Autodesk Inventor part; units mm, degrees
ref_plane "YZ Plane" through (0, 0, 0) normal (1, 0, 0) x (0, 1, 0)
ref_plane "XZ Plane" through (0, 0, 0) normal (0, 1, 0) x (-1, 0, 0)
ref_plane "XY Plane" through (0, 0, 0) normal (0, 0, 1) x (1, 0, 0)
sketch "Эскиз1" plane through (0, 0, 0) normal (1, 0, 0) x (0, 1, 0)
  circle A0 centre (0, 0) radius 4
  circle A1 centre (0, 0) radius 5
  line L0 (0, 5) -> (-2, 5)
  line L1 (-2, 5) -> (-2, 10)
  line L2 (-2, 10) -> (0, 10)
  line L3 (0, 10) -> (0, 5)
  line L4 (0, -5) -> (-2, -5)
  line L5 (-2, -5) -> (-2, -10)
  line L6 (-2, -10) -> (0, -10)
  line L7 (0, -10) -> (0, -5)
  line L8 (-2, 5) -> (-2, -5)
  line L9 (0, 5) -> (-2, 4.5826)
  line L10 (-2, -4.5826) -> (0, -5)
  line L11 (-2, 2) -> (-1, 3.873)
  line L12 (-2, -2) -> (-1, -3.873)
  line L13 (-1, -3.873) -> (-2, -3.873)
  line L14 (-1, 3.873) -> (-2, 3.873)
  dimension "d0" = 8
  dimension "d1" = 10
  dimension "d2" = 3
  dimension "d3" = 3
extrude "Выдавливание1" add sketch "Эскиз1" along normal blind 8 contours A0 L14 L8 L9 A1 L10 L13 | L11 L8 A0 | A0 L8 L14 | L13 L8 A0 | A0 L8 L12 | L8 L0 A1 | A1 L9 | L10 A1 | A1 L4 L8 | L0 L1 L2 L3 | L7 L6 L5 L4
fillet "Сопряжение2" radius 1.25 2 edges at (4, 0, 10) (4, 0, -10)
fillet "Сопряжение3" radius 1.5 2 edges at (4, -1, -3.873) (4, -1, 3.873)
sketch "Эскиз5" plane through (8, 0, 0) normal (1, 0, 0) x (0, 0, -1)
  circle A0 centre (0, 0) radius 5
  circle A1 centre (0, 0) radius 6
  line L0 (-5, 0) -> (-8.75, 0)
  line L1 (-6, 0) -> (-5, 0)
  arc A2 (5, 0) -> (-5, 0) centre (0, 0) ccw
  line L2 (-5, 0) -> (5, 0)
  line L3 (8.75, 0) -> (5, 0)
  line L4 (6, 0) -> (5, 0)
  dimension "d28" = 12
extrude "Выдавливание5" add sketch "Эскиз5" against normal blind 8 contours A0 L0 A1 L3 picked at (-5.5601, 0.8775)
fillet "Сопряжение4" radius 2.5 2 edges at (4, 0, 6) (4, 0, -6)
properties part number "binding links"
Verification items for the finished model (mm, model axes). A direction names the side the tool comes from. Round coordinates to 2 decimals unless told otherwise and drop trailing zeros. Order: outer loops, then holes, each group sorted by start corner. A loop starts at its lowest first (then second) coordinate and runs counter-clockwise, first axis right, second up. Notation, with made-up numbers: (49.5, 22.5) -> (65.5, 22.5) arc R26 ccw to (65.5, 46.5) -> close; hole circle Ø3 at (60.5, 19). An arc over 180 degrees is marked (long way). Put each result on its own line as item: value. Start each with the question number.
(1) Section check A-A (y = 3.5). Enter the section's corners in (x, z).
(2) Section check C-C (x = 5.5). Enter the section's corners in (y, z), then the cut area to 3 significant figures.
(3) Depth check by flat-ended pin: pin 1 Ø1 at (y, z) = (-0.5, 1.5) entering from +X; pin 2 Ø4 at (x, y) = (3, 4) entering from +Z; pin 3 Ø1 at (x, y) = (6.5, 3.5) entering from -Z. Enter the tip coordinate at first touch or a pass-through.
(4) Tool access check on faces 4 (the face through (4, 6, 0)), 5 (the face through (3.944, -1.682, -2.595)). Record the directions out of +Z, -Z, +X, -X, +Y, -Y that give a thin tool (end or side, any length) a straight path to the whole face; none if there is none.
(5) Section check B-B (z = 3.5). Enter the section's corners in (x, y), then the cut area to 3 significant figures.
(6) Section check D-D (z = 0). Enter the section's corners in (x, y).
(7) Draft check along Y on faces 1 (the face through (4, 4, 0)), 2 (the face through (4.056, -0.376, -9.644)), 3 (the face through (4, -2, 6)). Enter one of: +Y half, -Y half, draft (parallel to the pull), parting line (faces both ways), or undercut.
(8) Material ranges on line 1 along Y through (x, z) = (2.75, -8.75); line 2 along Y through (x, z) = (6.25, 0); line 3 along Y through (x, z) = (4.25, -3.5), recorded low to high.
Completed:
1. outline: (0, -4.87) -> (8, -4.87) -> (8, -1.94) -> (0, -1.94) -> close; (0, 1.94) -> (8, 1.94) -> (8, 4.87) -> (0, 4.87) -> close
2. outline: (-2, -10) -> (-1.25, -10) arc R1.25 ccw to (0, -8.75) -> (0, -8.12) arc R2.5 cw to (1.76, -5.73) arc R6 ccw to (1.76, 5.73) arc R2.5 cw to (0, 8.12) -> (0, 8.75) arc R1.25 ccw to (-1.25, 10) -> (-2, 10) -> (-2, 2) -> (-1.36, 3.21) arc R1.5 cw to (-0.05, 4) arc R4 cw (long way) to (-0.05, -4) arc R1.5 cw to (-1.36, -3.21) -> (-2, -2) -> close
2. area: 58.8 mm2
3. pin 1: passes through
3. pin 2: stops at z = 5.66
3. pin 3: stops at z = -5.2
4. face 4: +X, -X, +Y
4. face 5: +X, -X
5. outline: (0, -2) -> (8, -2) -> (8, -1.15) -> (0, -1.15) -> close; (0, 1.94) -> (8, 1.94) -> (8, 4.87) -> (0, 4.87) -> close
5. area: 30.3 mm2
6. outline: (0, 4) -> (8, 4) -> (8, 6) -> (0, 6) -> close
7. face 1: undercut
7. face 2: +Y half
7. face 3: -Y half
8. line 1: y = -2 to 0
8. line 2: y = 4 to 6
8. line 3: y = -2 to -1.15, 1.94 to 4.87
